Could you check a few things on this model? Use its own coordinates, in mm. Face numbers are marked on the shaded views. Coordinates: 2 decimals unless noted, no trailing zeros. Write each loop counter-clockwise with the first axis right and the second up, starting at its lowest first coordinate (ties: lowest second). Pieces come first, ordered by that corner, then holes.
Item 1: I want a section at B-B on z = -49.5. Please give me the cut outline in (x, y), then the cut area to 3 significant figures.
Item 2: I want a section at D-D on y = 0. Please give me the cut outline in (x, z), then the cut area to 3 significant figures.
Item 3: If I drill on probe 1 along X at (y, z) = (-5, -58.5); probe 2 along X at (y, z) = (-33, -75.5); probe 3 along Z at (x, y) = (-11, 38), over which ranges is the centre line in solid material (lowest first)?
Item 4: I want a section at C-C on x = -61. Please give me the cut outline in (y, z), then the cut area to 3 significant figures.
Item 5: I want a section at A-A on x = -8.5. Please give me the cut outline in (y, z), then the cut area to 3 significant figures.
Item 6: Thinking about a two-plate mould opening in Z: for the marked faces 1 and 2, which applies, +Z half, -Z half, draft (parallel to the pull), parting line (faces both ways), or undercut?
Item 7: For P1, Ø4, axis at x = -20.5, y = -19, coming from the +Z side; P2, Ø3.5, axis at y = 1, z = -33.5, coming from the +X side; P3, Ø3, axis at y = -39, z = -25, coming from the +X side, each with a flat end and sliding along its axis, tell me the tip position at first contact or that it passes through.
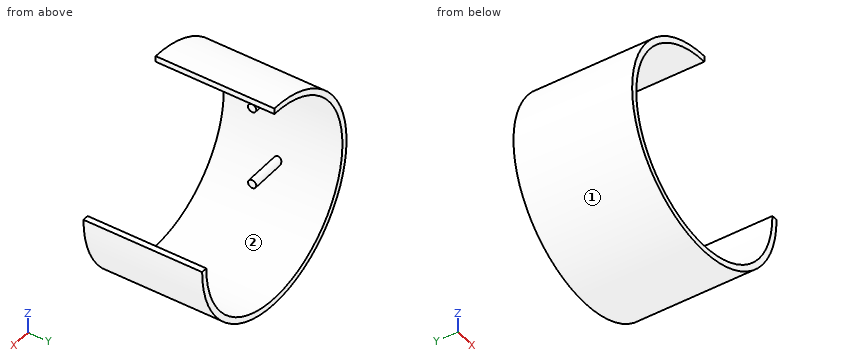
Autodesk Inventor part; units mm, degrees
ref_plane "YZ Plane" through (0, 0, 0) normal (1, 0, 0) x (0, 1, 0)
ref_plane "XZ Plane" through (0, 0, 0) normal (0, 1, 0) x (-1, 0, 0)
ref_plane "XY Plane" through (0, 0, 0) normal (0, 0, 1) x (1, 0, 0)
sketch "Sketch1" plane through (0, 0, 0) normal (0, 1, 0) x (-1, 0, 0)
  arc A0 (-87.5, 0) -> (0, 87.5) centre (0, 0) ccw
  arc A1 (-82.5, 0) -> (0, 82.5) centre (0, 0) ccw
  line L0 (0, 87.5) -> (0, 82.5)
  line L1 (-82.5, 0) -> (-87.5, 0)
  dimension "d0" = 165
  dimension "d1" = 175
  dimension "d7" = 0
  dimension "d8" = 0
extrude "Extrusion1" add sketch "Sketch1" along normal mid plane 100
sketch "Sketch3" plane through (0, 0, 0) normal (1, 0, 0) x (0, 1, 0)
  circle A0 centre (0, 34) radius 3.5
  circle A1 centre (0, -34) radius 3.5
  circle A2 centre (0, 34) radius 3.5
  circle A3 centre (0, -34) radius 3.5
  point P0 (0, 0)
  dimension "d9" = 7
  dimension "d10" = 7
  dimension "d11" = 68
  dimension "d12" = 34
  dimension "d13" = 34
extrude "Extrusion2" add sketch "Sketch3" against normal up to next
sketch "Sketch4" plane through (0, 0, 34) normal (1, 0, 0) x (0, 0, -1)
  circle A0 centre (0, 0) radius 3.5
  circle A1 centre (68, 0) radius 3.5
  circle A2 centre (68, 0) radius 3.5
  point P0 (34, 0)
extrude "Extrusion3" cut sketch "Sketch4" against normal blind 45
properties part number "airframe"
Response values:
1. outline: (-72.15, -50) - (-66, -50) - (-66, 50) - (-72.15, 50) - close; (66, -50) - (72.15, -50) - (72.15, 50) - (66, 50) - close
1. area: 1,230 mm2
2. outline: (-76.66, -30.5) arc R82.5 cw to (-76.66, 30.5) - (-45, 30.5) - (-45, 37.5) - (-73.48, 37.5) arc R82.5 cw to (0, 82.5) - (0, 87.5) arc R87.5 ccw (long way) to (87.5, 0) - (82.5, 0) arc R82.5 cw to (-73.48, -37.5) - (-45, -37.5) - (-45, -30.5) - close
2. area: 2,420 mm2
3. probe 1: x = -65.07 to -58.17, 58.17 to 65.07
3. probe 2: x = -44.23 to -33.26, 33.26 to 44.23
3. probe 3: z = -86.81 to -81.76, 81.76 to 86.81
4. outline: (-50, -62.73) - (50, -62.73) - (50, -55.55) - (-50, -55.55) - close; (-50, 55.55) - (50, 55.55) - (50, 62.73) - (-50, 62.73) - close; circle Ø7 at (0, -34); circle Ø7 at (0, 34)
4. area: 1,510 mm2
5. outline: (-50, -87.09) - (50, -87.09) - (50, -82.06) - (-50, -82.06) - close; (-50, 82.06) - (50, 82.06) - (50, 87.09) - (-50, 87.09) - close
5. area: 1,010 mm2
6. face 1: parting line
6. face 2: undercut
7. P1: stops at z = 85.52
7. P2: stops at x = 81.54
7. P3: stops at x = 84.29
